Design review of the part built by this model. Coordinates are the model's own, in mm. A direction names the side the tool comes from. Round coordinates to 2 decimals unless told otherwise and drop trailing zeros. Loops run counter-clockwise (first coordinate to the right, second up) from the corner with the lowest first, then second, coordinate; pieces in that order, holes last. Notation, with made-up numbers: (42, -27) - (74, -27) arc R12 ccw to (74, -8) - close; hole circle Ø11 at (6, 26). An arc over 180 degrees is marked (long way). Return JSON: item names as keys, results as strings. Group by question number.
from build123d import *

# Parameters (mm, degrees)
BOSS_EXTRUDE1_DEPTH = 1.5
SKETCH2_R           = 2.75
BOSS_EXTRUDE2_DEPTH = 6
SKETCH3_W           = 1.1
SKETCH3_H           = 1.45
SKETCH3_W_2         = 1.45
SKETCH3_H_2         = 1.1
CUT_EXTRUDE1_DEPTH  = 6
CHAMFER1_SIZE       = 0.3
FILLET1_R           = 1
SKETCH4_R           = 1.25
BOSS_EXTRUDE3_DEPTH = 0.01
DOME2_FACE_RADIUS   = 1.25
DOME2_HEIGHT        = 1.25
DOME3_FACE_RADIUS   = 1.25
DOME3_HEIGHT        = 1.25
DOME4_FACE_RADIUS   = 1.25
DOME4_HEIGHT        = 1.25
DOME6_FACE_RADIUS   = 1.25
DOME6_HEIGHT        = 1.25
FILLET3_R           = 0.2


with BuildPart() as part:
    # Sketch1 → Boss-Extrude1 (new body)
    with BuildSketch(Plane(origin=(0, 0, 0), x_dir=(1, 0, 0), z_dir=(0, 1, 0))):
        with BuildLine():
            Line((-7.324675649, 4.396717546), (4.675324351, 4.396717546))
            ThreePointArc((4.675324351, 4.396717546), (5.382431132, 4.103824327), (5.675324351, 3.396717546))
            Line((5.675324351, 3.396717546), (5.675324351, -8.603282454))
            ThreePointArc((5.675324351, -8.603282454), (5.382431132, -9.310389235), (4.675324351, -9.603282454))
            Line((4.675324351, -9.603282454), (-7.324675649, -9.603282454))
            ThreePointArc((-7.324675649, -9.603282454), (-8.03178243, -9.310389235), (-8.324675649, -8.603282454))
            Line((-8.324675649, -8.603282454), (-8.324675649, 3.396717546))
            ThreePointArc((-8.324675649, 3.396717546), (-8.03178243, 4.103824327), (-7.324675649, 4.396717546))
        make_face()
    extrude(amount=BOSS_EXTRUDE1_DEPTH)

    # Sketch2 → Boss-Extrude2 (add)
    with BuildSketch(Plane.XZ):
        with Locations(Location((-1.324675649, 2.603282454, 0), (0, 0, 270))):
            Circle(SKETCH2_R)
    extrude(amount=BOSS_EXTRUDE2_DEPTH)

    # Sketch3 → Cut-Extrude1 (cut)
    with BuildSketch(Plane.XZ.offset(6)):
        with Locations((-1.324675649, 3.878282454)):
            Rectangle(SKETCH3_W, SKETCH3_H)
        with Locations((-0.049675649, 2.603282454)):
            Rectangle(SKETCH3_W_2, SKETCH3_H_2)
        with Locations((-1.324675649, 2.603282454)):
            Rectangle(SKETCH3_W, SKETCH3_H_2)
        with Locations((-2.599675649, 2.603282454)):
            Rectangle(SKETCH3_W_2, SKETCH3_H_2)
        with Locations((-1.324675649, 1.328282454)):
            Rectangle(SKETCH3_W, SKETCH3_H)
    extrude(amount=-CUT_EXTRUDE1_DEPTH, mode=Mode.SUBTRACT)

    # Chamfer1
    chamfer1_edges = [part.edges().sort_by_distance(p)[0] for p in [
        (-0.774675649, -6, 3.878282454),
        (-0.049675649, -6, 3.153282454),
        (0.675324351, -6, 2.603282454),
        (-0.774675649, -6, 1.328282454),
        (-2.599675649, -6, 3.153282454),
        (-1.324675649, -6, 4.603282454),
        (-1.874675649, -6, 3.878282454),
        (-3.324675649, -6, 2.603282454),
        (-2.599675649, -6, 2.053282454),
        (-1.874675649, -6, 1.328282454),
        (-1.324675649, -6, 0.603282454),
        (-0.049675649, -6, 2.053282454),
    ]]
    chamfer(chamfer1_edges, length=CHAMFER1_SIZE)

    # Fillet1
    fillet1_edges = [part.edges().sort_by_distance(p)[0] for p in [
        (-1.324675649, 0, 5.353282454),
    ]]
    fillet(fillet1_edges, radius=FILLET1_R)

    # Sketch4 → Boss-Extrude3 (add)
    with BuildSketch(Plane(origin=(0, 1.5, 0), x_dir=(1, 0, 0), z_dir=(0, 1, 0))):
        with Locations(Location((0.675324351, -2.603282454, 0), (0, 0, 90))):
            Circle(SKETCH4_R)
        with Locations(Location((-3.324675649, -2.603282454, 0), (0, 0, 90))):
            Circle(SKETCH4_R)
        with Locations(Location((0.675324351, -6.603282454, 0), (0, 0, 90))):
            Circle(SKETCH4_R)
        with Locations(Location((0.675324351, 1.396717546, 0), (0, 0, 90))):
            Circle(SKETCH4_R)
    extrude(amount=BOSS_EXTRUDE3_DEPTH)

    # Dome2: a dome of height H over a round flat face of radius A is a cap of a sphere of radius (A * A + H * H) / (2 * H)
    dome2_r = (DOME2_FACE_RADIUS * DOME2_FACE_RADIUS + DOME2_HEIGHT * DOME2_HEIGHT) / (2 * DOME2_HEIGHT)
    dome2_base = Plane((0.675324351, 1.51, -1.396717546), z_dir=(0, 1, 0))
    with Locations(dome2_base.offset(DOME2_HEIGHT - dome2_r)):
        dome2_ball = Sphere(dome2_r, mode=Mode.PRIVATE)
    add(split(dome2_ball, bisect_by=dome2_base, keep=Keep.TOP, mode=Mode.PRIVATE))

    # Dome3: a dome of height H over a round flat face of radius A is a cap of a sphere of radius (A * A + H * H) / (2 * H)
    dome3_r = (DOME3_FACE_RADIUS * DOME3_FACE_RADIUS + DOME3_HEIGHT * DOME3_HEIGHT) / (2 * DOME3_HEIGHT)
    dome3_base = Plane((-3.324675649, 1.51, 2.603282454), z_dir=(0, 1, 0))
    with Locations(dome3_base.offset(DOME3_HEIGHT - dome3_r)):
        dome3_ball = Sphere(dome3_r, mode=Mode.PRIVATE)
    add(split(dome3_ball, bisect_by=dome3_base, keep=Keep.TOP, mode=Mode.PRIVATE))

    # Dome4: a dome of height H over a round flat face of radius A is a cap of a sphere of radius (A * A + H * H) / (2 * H)
    dome4_r = (DOME4_FACE_RADIUS * DOME4_FACE_RADIUS + DOME4_HEIGHT * DOME4_HEIGHT) / (2 * DOME4_HEIGHT)
    dome4_base = Plane((0.675324351, 1.51, 2.603282454), z_dir=(0, 1, 0))
    with Locations(dome4_base.offset(DOME4_HEIGHT - dome4_r)):
        dome4_ball = Sphere(dome4_r, mode=Mode.PRIVATE)
    add(split(dome4_ball, bisect_by=dome4_base, keep=Keep.TOP, mode=Mode.PRIVATE))

    # Dome6: a dome of height H over a round flat face of radius A is a cap of a sphere of radius (A * A + H * H) / (2 * H)
    dome6_r = (DOME6_FACE_RADIUS * DOME6_FACE_RADIUS + DOME6_HEIGHT * DOME6_HEIGHT) / (2 * DOME6_HEIGHT)
    dome6_base = Plane((0.675324351, 1.51, 6.603282454), z_dir=(0, 1, 0))
    with Locations(dome6_base.offset(DOME6_HEIGHT - dome6_r)):
        dome6_ball = Sphere(dome6_r, mode=Mode.PRIVATE)
    add(split(dome6_ball, bisect_by=dome6_base, keep=Keep.TOP, mode=Mode.PRIVATE))

    # Fillet3
    fillet3_edges = [part.edges().sort_by_distance(p)[0] for p in [
        (5.382431132, 1.5, 9.310389235),
        (-1.324675649, 0, 9.603282454),
        (-8.03178243, 0, 9.310389235),
        (5.675324351, 1.5, 2.603282454),
        (5.382431132, 1.5, -4.103824327),
        (-1.324675649, 1.5, -4.396717546),
        (-8.03178243, 1.5, -4.103824327),
        (-8.324675649, 1.5, 2.603282454),
        (-8.03178243, 1.5, 9.310389235),
        (-1.324675649, 1.5, 9.603282454),
        (-8.324675649, 0, 2.603282454),
        (-8.03178243, 0, -4.103824327),
        (-1.324675649, 0, -4.396717546),
        (5.382431132, 0, -4.103824327),
        (5.675324351, 0, 2.603282454),
        (5.382431132, 0, 9.310389235),
    ]]
    fillet(fillet3_edges, radius=FILLET3_R)


solid = part.part
Q1. Add section D-D, the plane y = 2. State the section outline as (x, z) points.
Q2. Tool access review of faces 4 (the flat face through (2, 0, 6)), 5 (the cylindrical face through (5.39, 0.74, 9.3)), 6 (the flat face through (-1, 1.5, 3)): name each direction out of +Z, -Z, +X, -X, +Y, -Y from which nothing blocks a thin tool from reaching the whole face with its end or side.
Q3. Add section B-B, the plane z = -3. State the section outline as (x, y) points.
Q4. Add section C-C, the plane y = -2.75. State the section outline as (x, z) points, plus the area to 3 significant figures.
Q5. Insertion check: pin 1 Ø1.2 at (y, z) = (-2, 1.5) entering from +X; pin 2 Ø1 at (x, y) = (-1, -1.5) entering from +Z; pin 3 Ø0.7 at (x, y) = (-3, -2.5) entering from -Z. Each pin has a flat end and moves straight along its axis. Give the tip position at first contact, or say it passes through.
Q6. Add section A-A, the plane x = -6.5. State the section outline as (y, z) points.
Q7. For line 1 (Y direction, x = -1.25, z = -2); line 2 (X direction, y = -5.25, z = 1.75); line 3 (Z direction, x = -2.75, y = -3.25), list the stretches that pass through material, from the lowest coordinate up.
Q8. Draft analysis for pull direction Z (two halves, no side actions). For faces 1 (the flat face through (-1.875, -3, 4)), 2 (the flat face through (-3, -6, 1)), 3 (the cylindrical face through (-8.04, 0.742, -4.096)), state which applies: pulls with the +Z half, pulls with the -Z half, needs draft (parallel to the pull), parting line crosses it, or undercut.
Evaluation:
{
 "1": {"outline": "circle Ø2.3 at (-3.32, 2.6); circle Ø2.3 at (0.68, -1.4); circle Ø2.3 at (0.68, 2.6); circle Ø2.3 at (0.68, 6.6)"},
 "2": {"face 4": "-Y", "face 5": "+Z, +X, +Y, -Y", "face 6": "+Y"},
 "3": {"outline": "(-8.32, 0.2) arc R0.2 ccw to (-8.12, 0) - (5.48, 0) arc R0.2 ccw to (5.68, 0.2) - (5.68, 1.3) arc R0.2 ccw to (5.48, 1.5) - (-8.12, 1.5) arc R0.2 ccw to (-8.32, 1.3) - close"},
 "4": {"outline": "circle Ø5.5 at (-1.32, 2.6); hole (-3.32, 2.05) - (-1.87, 2.05) - (-1.87, 0.6) - (-0.77, 0.6) - (-0.77, 2.05) - (0.68, 2.05) - (0.68, 3.15) - (-0.77, 3.15) - (-0.77, 4.6) - (-1.87, 4.6) - (-1.87, 3.15) - (-3.32, 3.15) - close", "area": "16.2 mm²"},
 "5": {"pin 1": "x = 1.38", "pin 2": "z = 5.35", "pin 3": "z = 0.19"},
 "6": {"outline": "(0, -4.2) arc R0.2 ccw to (0.2, -4.4) - (1.3, -4.4) arc R0.2 ccw to (1.5, -4.2) - (1.5, 9.4) arc R0.2 ccw to (1.3, 9.6) - (0.2, 9.6) arc R0.2 ccw to (0, 9.4) - close"},
 "7": {"line 1": "0 to 1.5", "line 2": "-3.94 to -1.87, -0.77 to 1.29", "line 3": "0.25 to 2.05, 3.15 to 4.96"},
 "8": {"face 1": "undercut", "face 2": "needs draft", "face 3": "pulls with the -Z half"}
}
